Here's how the part is built. I have some questions about the finished solid (model axes, mm). A direction names the side the tool comes from. Coordinates: 2 decimals unless noted, no trailing zeros. Write each loop counter-clockwise with the first axis right and the second up, starting at its lowest first coordinate (ties: lowest second). Pieces come first, ordered by that corner, then holes.
Item 1: I want a section at B-B (x = 15.75). Please give me the cut outline in (y, z), and give its area (3 significant figures).
Item 2: I'm going to push flat-ended pins straight in: P1, Ø1.7, axis at y = 13, z = -0.5, coming from the +X side; P2, Ø1.5, axis at x = 10.5, z = 6.5, coming from the -Y side; P3, Ø1, axis at x = 7, z = -10, coming from the -Y side. Where does each tip first touch, or does it pass through?
Item 3: For faces 1 (the face through (17.475, -5, 3)), 2 (the face through (11.125, -13, 0)), 3 (the face through (7.925, 0, 5)), 4 (the face through (11.125, 13, 0)), 5 (the face through (6.35, 14, -8)), which set-ups out of +Z, -Z, +X, -X, +Y, -Y let a thin tool reach every point of the face, with its end or its side?
Item 4: Please list where these lines run through material, in increasing order: line 1 (Z direction, x = 3.5, y = 0); line 2 (Z direction, x = 6, y = 0).
Item 5: If we mould it in two halves opening along Y, with no side actions, what happens to faces 6 (the face through (17.35, 0.17, -16.21)), 7 (the face through (14, 11.055, 0)), 8 (the face through (5.592, -1.953, -14.877))? For each: pulls with the +Y half, pulls with the -Y half, needs draft (parallel to the pull), parting line crosses it, or undercut.
Item 6: I want a section at C-C (x = 10.5). Please give me the cut outline in (y, z), and give its area (4 significant figures).
Item 7: I want a section at A-A (x = 2.75). Please give me the cut outline in (y, z) (1 decimal).
from build123d import *

# Parameters (mm, degrees)
SKETCH3_W          = 134.7724
SKETCH3_H          = 67.3862
SKETCH3_W_2        = 67.3862
SKETCH3_H_2        = 22.1107
CUT_EXTRUDE1_DEPTH = 6.35
SKETCH4_W          = 7.9248
SKETCH4_H          = 11.1125


with BuildPart() as part:
    # Sketch1 → Revolve1 (revolve)
    with BuildSketch(Plane.XY):
        Polygon((0, 0), (0, 15.25905), (0.762, 16.02105), (4.318, 16.02105), (5.334, 15.00505), (6.35, 15.00505), (6.35, 16.84655), (16.7132, 16.84655), (17.4752, 16.08455), (17.4752, 0), align=None)
    revolve(axis=Axis((17.4752, 0, 0), (-1, 0, 0)))

    # Sketch2 → Cut-Revolve1 (revolve, cut)
    with BuildSketch(Plane.XY):
        Polygon((0, 0), (0, 4.3688), (2.398876108, 4.3688), (16.840187191, 4.819651116), (17.4752, 5.454663925), (17.4752, 0), align=None)
    revolve(axis=Axis((17.4752, 0, 0), (-1, 0, 0)), mode=Mode.SUBTRACT)

    # Sketch3 → Cut-Extrude1 (cut)
    with BuildSketch(Plane(origin=(17.4752, 0, 0), x_dir=(0, 0, -1), z_dir=(1, 0, 0))):
        Rectangle(SKETCH3_W, SKETCH3_H)
        Rectangle(SKETCH3_W_2, SKETCH3_H_2, mode=Mode.SUBTRACT)
    extrude(amount=-CUT_EXTRUDE1_DEPTH, mode=Mode.SUBTRACT)

    # Sketch4 → Cut-Revolve2 (revolve, cut)
    with BuildSketch(Plane.XY):
        with Locations((3.9624, 5.55625)):
            Rectangle(SKETCH4_W, SKETCH4_H)
    revolve(axis=Axis((7.9248, 0, 0), (-1, 0, 0)), mode=Mode.SUBTRACT)

    # Sketch5 → Revolve2 (revolve)
    with BuildSketch(Plane.XY):
        with BuildLine():
            Line((5.013509175, 16.762381804), (6.216617928, 15.559273051))
            ThreePointArc((6.216617928, 15.559273051), (6.253815367, 15.46947049), (6.216617928, 15.379667928))
            Line((6.216617928, 15.379667928), (5.842, 15.00505))
            Line((5.842, 15.00505), (5.334, 15.00505))
            Line((5.334, 15.00505), (5.334, 14.75105))
            Line((5.334, 14.75105), (6.35, 14.75105))
            Line((6.35, 14.75105), (6.35, 15.713259175))
            Line((6.35, 15.713259175), (5.216709175, 16.84655))
            Line((5.216709175, 16.84655), (5.013509175, 16.84655))
            Line((5.013509175, 16.84655), (5.013509175, 16.762381804))
        make_face()
    revolve(axis=Axis((6.35, 0, 0), (-1, 0, 0)))


solid = part.part
Answer:
1. outline: (-11.06, -12.71) arc R16.85 ccw to (11.06, -12.71) - (11.06, 12.71) arc R16.85 ccw to (-11.06, 12.71) - close; hole circle Ø9.57 at (0, 0)
1. area: 615 mm2
2. P1: stops at x = 11.13
2. P2: stops at y = -15.83
2. P3: stops at y = -13.91
3. face 1: +Z, -Z, +X, +Y, -Y
3. face 2: +Z, -Z, +X, -Y
3. face 3: -X
3. face 4: +Z, -Z, +X, +Y
3. face 5: none
4. line 1: z = -16.02 to -11.11, 11.11 to 16.02
4. line 2: z = -16.06 to -15.78, -15.16 to -11.11, 11.11 to 15.16, 15.78 to 16.06
5. face 6: parting line crosses it
5. face 7: pulls with the +Y half
5. face 8: undercut
6. outline: circle Ø33.69 at (0, 0); hole circle Ø9.24 at (0, 0)
6. area: 824.5 mm2
7. outline: circle Ø32 at (0, 0); hole circle Ø22.2 at (0, 0)
